The listing builds one solid part. Answer for the finished solid, in the listing's coordinates (mm). Face numbers are marked on the shaded views. A direction names the side the tool comes from. Coordinates: 2 decimals unless noted, no trailing zeros. Order: outer loops, then holes, each group sorted by start corner. A loop starts at its lowest first (then second) coordinate and runs counter-clockwise, first axis right, second up. Notation, with made-up numbers: (83, 87.25) - (98, 87.25) arc R22 ccw to (98, 97.25) - close; hole circle Ø1 at (-9, 32). An arc over 180 degrees is marked (long way). Use a Markdown table: item, result. Add a question column.
Item 1: The part is cut by section A-A, the plane x = 0. Give the vertices of the cut face in (y, z), then the cut area to 3 significant figures.
Item 2: For the marked faces 1 and 2, determine the directions among +Z, -Z, +X, -X, +Y, -Y from which every point of the face is accessible in a straight line to the end or side of a thin tool.
Item 3: Flat-ended cylindrical pins translate along their axes: P1, Ø3, axis at y = 1, z = -4, coming from the +X side; P2, Ø1, axis at x = 1, z = -7.5, coming from the +Y side; P3, Ø1.5, axis at x = -1, z = -6, coming from the +Y side. Find the tip coordinate at first contact, or state that the pin passes through.
Item 4: Find the intervals of material crossed by line 1 along Z through (x, y) = (-1.7, 1.95); line 2 along Z through (x, y) = (0.7, -1.1); line 3 along X through (y, z) = (-0.55, -11), in increasing order.
Item 5: The part is cut by section C-C, the plane z = -7.75. Give the vertices of the cut face in (x, y), then the cut area to 3 significant figures.
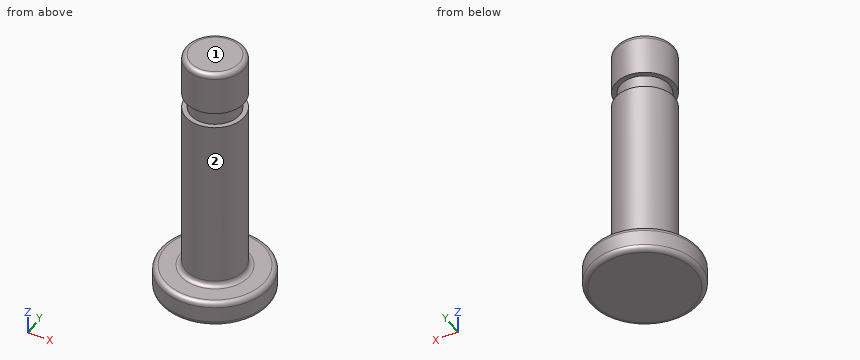
from build123d import *

# Parameters (mm, degrees)
FILLET_1_R = 0.25


with BuildPart() as part:
    # 草图1 → 旋转1 (revolve)
    with BuildSketch(Plane.YZ, mode=Mode.PRIVATE) as revolve_1_sk:
        Polygon((0, 0), (-1.5, 0), (-1.5, -2.2), (-1.25, -2.2), (-1.25, -3), (-1.5, -3), (-1.5, -12), (-2.8, -12), (-2.8, -13.3), (0, -13.3), align=None)
    revolve(revolve_1_sk.sketch.rotate(Axis((0, 0, -13.3), (0, 0, 1)), 180), axis=Axis((0, 0, -13.3), (0, 0, 1)))

    # 圆角1
    fillet_1_edges = [part.edges().sort_by_distance(p)[0] for p in [
        (0, -1.5, 0),
        (0, -2.8, -13.3),
        (0, -2.8, -12),
        (0, -1.5, -12),
    ]]
    fillet(fillet_1_edges, radius=FILLET_1_R)


solid = part.part
Solution:
| question | item | result |
|---|---|---|
| 1 | outline | (-2.8, -13.05) arc R0.25 ccw to (-2.55, -13.3) - (2.55, -13.3) arc R0.25 ccw to (2.8, -13.05) - (2.8, -12.25) arc R0.25 ccw to (2.55, -12) - (1.75, -12) arc R0.25 cw to (1.5, -11.75) - (1.5, -3) - (1.25, -3) - (1.25, -2.2) - (1.5, -2.2) - (1.5, -0.25) arc R0.25 ccw to (1.25, 0) - (-1.25, 0) arc R0.25 ccw to (-1.5, -0.25) - (-1.5, -2.2) - (-1.25, -2.2) - (-1.25, -3) - (-1.5, -3) - (-1.5, -11.75) arc R0.25 cw to (-1.75, -12) - (-2.55, -12) arc R0.25 ccw to (-2.8, -12.25) - close |
| 1 | area | 42.8 mm2 |
| 2 | face 1 | +Z, +X, -X, +Y, -Y |
| 2 | face 2 | +Z |
| 3 | P1 | stops at x = 1.5 |
| 3 | P2 | stops at y = 1.41 |
| 3 | P3 | stops at y = 1.48 |
| 4 | line 1 | z = -13.3 to -12 |
| 4 | line 2 | z = -13.3 to -3, -2.2 to -0.01 |
| 4 | line 3 | x = -1.4 to 1.4 |
| 5 | outline | circle Ø3 at (0, 0) |
| 5 | area | 7.07 mm2 |
